from build123d import *

# Parameters (mm, degrees)
SKETCH1_R                           = 7.9375
BOSS_EXTRUDE1_DEPTH                 = 76.2
F_1_8_0_1250_DOWEL_HOLE1_D          = 3.175
F_1_8_0_1250_DOWEL_HOLE1_DEPTH      = 17.526
F_1_8_0_1250_DOWEL_HOLE1_TIP        = 0.953866233
F_5_0MM_DOWEL_HOLE1_D               = 5
F_5_0MM_DOWEL_HOLE1_DEPTH           = 25.4
F_5_0MM_DOWEL_HOLE1_TIP             = 1.502151548
TAP_DRILL_FOR_1_4_20_TAP1_OUTLINE_R = 2.5527
TAP_DRILL_FOR_1_4_20_TAP1_DEPTH     = 9


with BuildPart() as part:
    # Sketch1 → Boss-Extrude1 (new body)
    with BuildSketch(Plane(origin=(0, 0, 0), x_dir=(1, 0, 0), z_dir=(0, 1, 0))):
        with Locations(Location((0, 0, 0), (0, 0, 90))):
            Circle(SKETCH1_R)
    extrude(amount=BOSS_EXTRUDE1_DEPTH)

    # 1/8 (0.1250) Dowel Hole1
    with Locations(Plane(origin=(6.688476845, 68.670007772, -4.274129589), x_dir=(0.538473019062, 0, 0.842642752145), z_dir=(0.842642752145, 0, -0.538473019062))):
        with Locations((0, 0)):
            Hole(F_1_8_0_1250_DOWEL_HOLE1_D / 2, depth=F_1_8_0_1250_DOWEL_HOLE1_DEPTH)
            with Locations((0, 0, -(F_1_8_0_1250_DOWEL_HOLE1_DEPTH + F_1_8_0_1250_DOWEL_HOLE1_TIP / 2))):  # 118° drill point
                Cone(0, F_1_8_0_1250_DOWEL_HOLE1_D / 2, F_1_8_0_1250_DOWEL_HOLE1_TIP, mode=Mode.SUBTRACT)

    # Ø5.0mm Dowel Hole1
    with Locations(Plane(origin=(0, 0, 0), x_dir=(-1, 0, 0), z_dir=(0, -1, 0))):
        with Locations((0, 0)):
            Hole(F_5_0MM_DOWEL_HOLE1_D / 2, depth=F_5_0MM_DOWEL_HOLE1_DEPTH)
            with Locations((0, 0, -(F_5_0MM_DOWEL_HOLE1_DEPTH + F_5_0MM_DOWEL_HOLE1_TIP / 2))):  # 118° drill point
                Cone(0, F_5_0MM_DOWEL_HOLE1_D / 2, F_5_0MM_DOWEL_HOLE1_TIP, mode=Mode.SUBTRACT)

    # Tap Drill for 1/4-20 Tap1: read off the stored shape, not the designer's step
    # Tap Drill for 1/4-20 Tap1 outline → Tap Drill for 1/4-20 Tap1 (cut)
    with BuildSketch(Plane(origin=(0, 0, 0), x_dir=(0, 1, 0), z_dir=(0.9087676630767977, 0, -0.4173024497243409))):
        with Locations((10.457639215, 0)):
            Circle(TAP_DRILL_FOR_1_4_20_TAP1_OUTLINE_R)
        with Locations((21.887639215, 0)):
            Circle(TAP_DRILL_FOR_1_4_20_TAP1_OUTLINE_R)
    extrude(amount=TAP_DRILL_FOR_1_4_20_TAP1_DEPTH, mode=Mode.SUBTRACT)


solid = part.part
Work out the finished part from the listing and answer in its coordinate system (mm). A direction names the side the tool comes from. Coordinates: 2 decimals unless noted, no trailing zeros. Write each loop counter-clockwise with the first axis right and the second up, starting at its lowest first coordinate (ties: lowest second). Pieces come first, ordered by that corner, then holes. Notation, with made-up numbers: M 63,-20.75 L 81,-20.75 A34 ccw 81,11.25 Z; hole C 57.5,-2.5 d10. An arc over 180 degrees is marked long. Use one line per item in the form item = value. Start each with the question number.
1. The part is cut by section C-C (z = -6.5). Give the vertices of the cut face in (x, y).
2. Each of these flat-tipped pins is pushed along its axis until it touches: P1, Ø4, axis at y = 65, z = -5, coming from the +X side; P2, Ø5, axis at x = 6, y = 36.5, coming from the -Z side; P3, Ø1.5, axis at x = -2, y = 52.5, coming from the +Z side. Where does it stop, or does it pass through?
3. The mould has two halves that part along Z. Classify faces 1 (the face through (-2, 0, 2)), 2 (the face through (3.71, 8.43, -3.41)), 3 (the face through (-5.365, 37.567, 5.85)): released by +Z, released by -Z, zero draft, split by the parting line, or undercut.
4. The part is cut by section A-A (y = 50.5). Give the vertices of the cut face in (x, z) (1 decimal), plus the area to 3 significant figures.
5. Straight lines are drawn through the part: probe 1 along X at (y, z) = (20.5, -0.5); probe 2 along Z at (x, y) = (0.25, 52.5); probe 3 along X at (y, z) = (14, -2.25). For each, find the intervals that lie inside material, in ascending order. Write a range as from..to.
6. A tool of negligible diameter and unlimited length cuts with its end or side. For faces 4 (the face through (0.09, 70.22, 0.35)), 5 (the face through (-2, 12.9, 1.5)), from which of +Z, -Z, +X, -X, +Y, -Y can it reach the whole face along a straight path? Write none if from no direction.
Evaluation:
q1.outline = M -4.56,0 L 4.56,0 L 4.56,76.2 L -4.56,76.2 Z
q2.P1 = 7.35
q2.P2 = -7.12
q2.P3 = 7.84
q3.face_1 = zero draft
q3.face_2 = undercut
q3.face_3 = split by the parting line
q4.outline = C 0,0 d15.9
q4.area = 198 mm^2
q5.probe_1 = -7.92..-2.45, 6.22..7.92
q5.probe_2 = -7.93..7.93
q5.probe_3 = -7.61..-1.09, 1.09..7.61
q6.face_4 = none
q6.face_5 = -Y
